The drawing under review shows one solid part. Ordinate dimensions are in mm from its lowest x, y, z. A direction names the side the tool comes from. Coordinates: 2 decimals unless noted, no trailing zeros. Order: outer loops, then holes, each group sorted by start corner. A loop starts at its lowest first (then second) coordinate and runs counter-clockwise, first axis right, second up. Notation, with made-up numbers: (-9, -36.75) - (33, -36.75) arc R15 ccw to (33, -30.75) - close; hole circle Ø1 at (72.25, 0). An arc over 180 degrees is marked (long way). Write item = value, one per line. Start each with the question number.
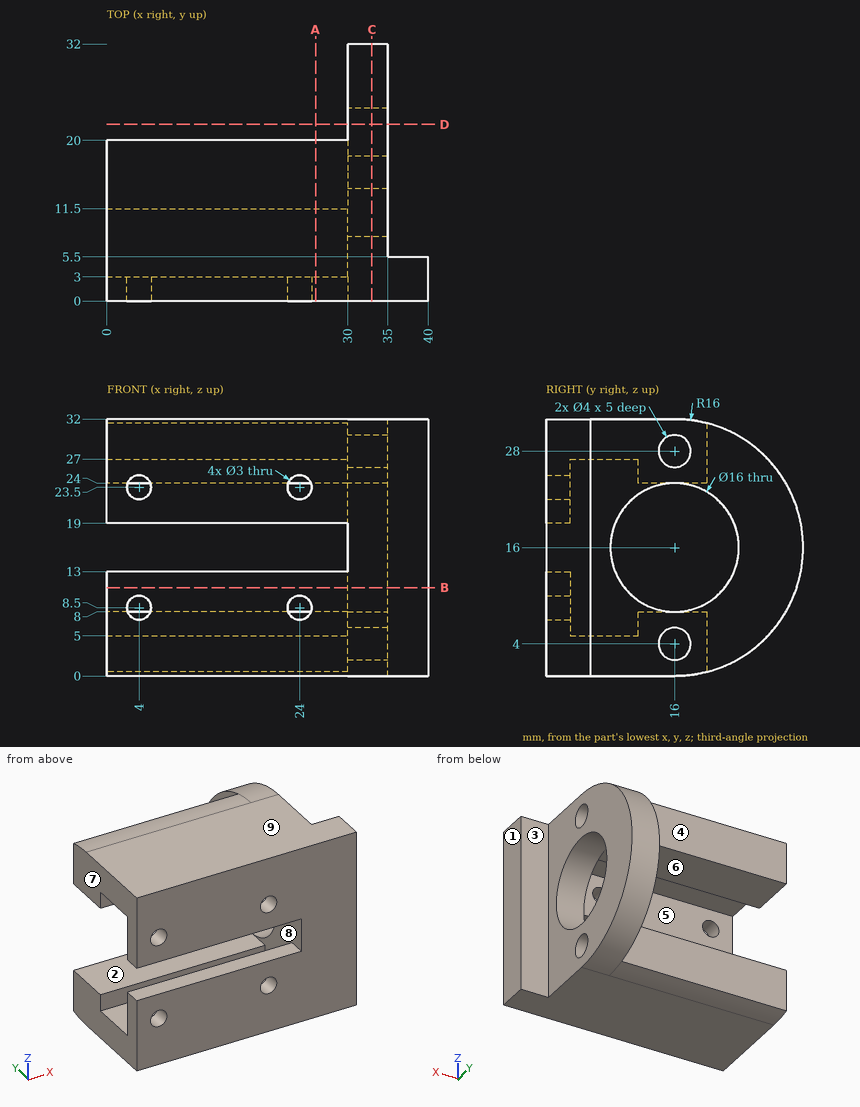
Item 1: Add section B-B on z = 11. Give the boundary of the cut face in (x, y) (3 decimals), plus the area to 3 significant figures.
Item 2: Add section A-A on x = 26. Give the boundary of the cut face in (y, z).
Item 3: For P1, Ø3.5, axis at x = 4, z = 8.5, coming from the +Y side; P2, Ø2.5, axis at x = 11, y = 5.5, coming from the -Z side; P3, Ø6, axis at y = 28, z = 14, coming from the -X side; P4, Ø1.5, axis at x = 28, z = 11, coming from the +Y side, all flat-tipped, find the tip position at first contact; note any pin that passes through.
Item 4: Add section C-C on x = 33. Give the boundary of the cut face in (y, z).
Item 5: Mouldability with a two-part tool opening along Z and no side actions: class the marked faces 6, 7, 8 and 9 as +Z half, -Z half, draft (parallel to the pull), parting line (faces both ways), or undercut.
Item 6: For line 1 (Z direction, x = 2.5, y = 13); line 2 (Z direction, x = 4, y = 1.3); line 3 (Y direction, x = 21.5, z = 6.5), list the stretches that pass through material, from the lowest coordinate up.
Item 7: Add section D-D on y = 22. Give the boundary of the cut face in (x, z).
Item 8: For the marked faces 1, 2, 3, 4 and 5, list the 3-axis set-ups (+Z, -Z, +X, -X, +Y, -Y) from which the entire face can be reached by the end or side of a thin tool; tool diameter is ignored.
Worked out:
q1.outline = (0, 0) - (40, 0) - (40, 5.5) - (35, 5.5) - (35, 9.755) - (30, 9.755) - (30, 3) - (0, 3) - close; (30, 22.245) - (35, 22.245) - (35, 31.199) - (30, 31.199) - close
q1.area = 211 mm2
q2.outline = (0, 0) - (16, 0) arc R16 ccw to (20, 0.51) - (20, 8) - (11.5, 8) - (11.5, 5) - (3, 5) - (3, 13) - (0, 13) - close; (0, 19) - (3, 19) - (3, 27) - (11.5, 27) - (11.5, 24) - (20, 24) - (20, 31.49) arc R16 ccw to (16, 32) - (0, 32) - close
q3.P1 = 20
q3.P2 = 0
q3.P3 = 30
q3.P4 = 3
q4.outline = (0, 0) - (16, 0) arc R16 ccw to (16, 32) - (0, 32) - close; hole circle Ø16 at (16, 16); hole circle Ø4 at (16, 4); hole circle Ø4 at (16, 28)
q5.face_6 = undercut
q5.face_7 = draft
q5.face_8 = undercut
q5.face_9 = +Z half
q6.line_1 = 0 to 8, 24 to 32
q6.line_2 = 0 to 7, 10 to 13, 19 to 22, 25 to 32
q6.line_3 = 0 to 3, 11.5 to 20
q7.outline = (30, 1.17) - (35, 1.17) - (35, 10.71) - (30, 10.71) - close; (30, 21.29) - (35, 21.29) - (35, 30.83) - (30, 30.83) - close
q8.face_1 = +Z, -Z, +X, +Y, -Y
q8.face_2 = -X, +Y
q8.face_3 = +Z, -Z, +X, +Y
q8.face_4 = +Z, -Z, -X, +Y
q8.face_5 = -X
